Geometry: final body of the model. Coordinates: model frame, mm. Face numbers are marked on the shaded views. A direction names the side the tool comes from. Give positions to 0.01 mm unless a question says otherwise; leave off trailing zeros. Write each loop counter-clockwise with the first axis right and the second up, starting at its lowest first coordinate (ties: lowest second). Pieces come first, ordered by that corner, then holes. Notation, with made-up numbers: M 83,83 L 129,83 A28 cw 129,108 Z; hole C 46,74.5 d2. An arc over 180 degrees is marked long. Use a Markdown table: item, result. Add a question column.
(1) Reachability of the marked faces 4 and 5 from +Z, -Z, +X, -X, +Y, -Y: full face, straight path, thin tool, end or side. Return the list, or none.
(2) Material intervals for L1, parallel to Y at x = 6.45, z = 15; L2, parallel to Y at x = -6.1, z = 5; L3, parallel to X at y = 0, z = 11.25, sorted ascending.
(3) Cut plane C-C (x = -13). Output: boundary loops of the cut face in (y, z).
(4) Cut plane A-A (z = 5). Output: boundary loops of the cut face in (x, y).
(5) Draft query along X for the marked faces 1, 2 and 3. Return one class per face: released by +X, released by -X, zero draft, split by the parting line, or undercut.
(6) Cut plane B-B (y = 8). Output: boundary loops of the cut face in (x, z), plus the area to 3 significant figures.
(7) Pin query (flat end, axial travel): pin 1 Ø2 at (x, z) = (0.5, 15.5) entering from +Y; pin 2 Ø3 at (x, z) = (-24, 9.5) entering from -Y; pin 3 Ø3 at (y, z) = (-2.5, 12.5) entering from +X. Return the tip coordinate at first contact, or that it passes through.
(8) Cut plane D-D (z = 10). Output: boundary loops of the cut face in (x, y).
```python
from build123d import *

# Parameters (mm, degrees)
EXTRUSION2_DEPTH = 20
ESQUISSE8_R      = 1.5
EXTRUSION3_DEPTH = 76.056550285
ESQUISSE9_R      = 1.5
EXTRUSION4_DEPTH = 76.056550285


with BuildPart() as part:
    # Esquisse7 → Extrusion2 (new body)
    with BuildSketch(Plane.XY):
        with BuildLine():
            Line((5.5, -57.037143518), (7.5, -57.037143518))
            Line((7.5, -57.037143518), (7.5, -37.037143518))
            ThreePointArc((7.5, -37.037143518), (7.717796634, -36.414120329), (8.276315789, -36.062481847))
            ThreePointArc((8.276315789, -36.062481847), (0, 37), (-8.276315789, -36.062481847))
            ThreePointArc((-8.276315789, -36.062481847), (-7.717796634, -36.414120329), (-7.5, -37.037143518))
            Line((-7.5, -37.037143518), (-7.5, -57.037143518))
            Line((-7.5, -57.037143518), (-5.5, -57.037143518))
            Line((-5.5, -57.037143518), (-5.5, -37.037143518))
            ThreePointArc((-5.5, -37.037143518), (-6.153389903, -35.16807395), (-7.828947368, -34.113158504))
            ThreePointArc((-7.828947368, -34.113158504), (0, 35), (7.828947368, -34.113158504))
            ThreePointArc((7.828947368, -34.113158504), (6.153389903, -35.16807395), (5.5, -37.037143518))
            Line((5.5, -37.037143518), (5.5, -57.037143518))
        make_face()
    extrude(amount=EXTRUSION2_DEPTH)

    # Esquisse8 → Extrusion3 (cut, through all)
    with BuildSketch(Plane.ZY.offset(7.5)):
        with Locations((15, -52.037143518)):
            Circle(ESQUISSE8_R)
    extrude(amount=-EXTRUSION3_DEPTH, mode=Mode.SUBTRACT)

    # Esquisse9 → Extrusion4 (cut, through all)
    with BuildSketch(Plane.ZY.offset(7.5)):
        with Locations((5, -42.037143518)):
            Circle(ESQUISSE9_R)
    extrude(amount=-EXTRUSION4_DEPTH, mode=Mode.SUBTRACT)


solid = part.part
```
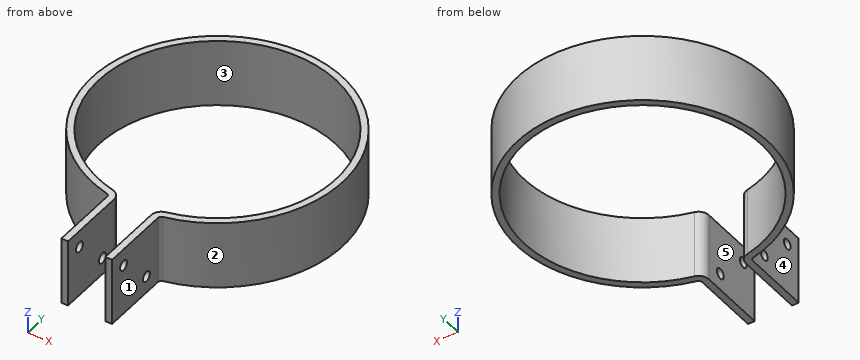
Answer list:
| question | item | result |
|---|---|---|
| 1 | face 4 | +Z, -Z, -X, -Y |
| 1 | face 5 | +Z, -Z, -Y |
| 2 | L1 | -57.04 to -53.54, -50.54 to -34.85, 34.4 to 36.43 |
| 2 | L2 | -57.04 to -43.54, -40.54 to -35.24, 34.46 to 36.49 |
| 2 | L3 | -37 to -35, 35 to 37 |
| 3 | outline | M -34.64,0 L -32.5,0 L -32.5,20 L -34.64,20 Z; M 32.5,0 L 34.64,0 L 34.64,20 L 32.5,20 Z |
| 4 | outline | M -8.28,-36.06 A1 cw -7.5,-37.04 L -7.5,-40.54 L -5.5,-40.54 L -5.5,-37.04 A3 ccw -7.83,-34.11 A35 cw long 7.83,-34.11 A3 ccw 5.5,-37.04 L 5.5,-40.54 L 7.5,-40.54 L 7.5,-37.04 A1 cw 8.28,-36.06 A37 ccw long Z; M -7.5,-57.04 L -5.5,-57.04 L -5.5,-43.54 L -7.5,-43.54 Z; M 5.5,-57.04 L 7.5,-57.04 L 7.5,-43.54 L 5.5,-43.54 Z |
| 5 | face 1 | released by +X |
| 5 | face 2 | split by the parting line |
| 5 | face 3 | undercut |
| 6 | outline | M -36.12,0 L -34.07,0 L -34.07,20 L -36.12,20 Z; M 34.07,0 L 36.12,0 L 36.12,20 L 34.07,20 Z |
| 6 | area | 82.1 mm² |
| 7 | pin 1 | y = 37 |
| 7 | pin 2 | y = -29.37 |
| 7 | pin 3 | x = 36.99 |
| 8 | outline | M -8.28,-36.06 A1 cw -7.5,-37.04 L -7.5,-57.04 L -5.5,-57.04 L -5.5,-37.04 A3 ccw -7.83,-34.11 A35 cw long 7.83,-34.11 A3 ccw 5.5,-37.04 L 5.5,-57.04 L 7.5,-57.04 L 7.5,-37.04 A1 cw 8.28,-36.06 A37 ccw long Z |
